Geometry: final body of the model. Coordinates: model frame, mm. Give positions to 0.01 mm unless a question says otherwise; leave off trailing zeros. Order: outer loops, then holes, each group sorted by start corner. A loop starts at its lowest first (then second) coordinate and runs counter-clockwise, first axis right, second up. Notation, with made-up numbers: (25.5, 10) - (56.5, 10) arc R17 ccw to (56.5, 16) - close; hole circle Ø5 at (80, -39). An arc over 180 degrees is marked (long way). One line per item, written item: value.
```python
from build123d import *

# Parameters (mm, degrees)
SKETCH1_W            = 20.5
SKETCH1_H            = 18.5
BOSS_EXTRUDE1_DEPTH  = 2
SKETCH2_W            = 2
SKETCH2_H            = 18.5
BOSS_EXTRUDE2_DEPTH  = 45
SKETCH4_W            = 20.5
SKETCH4_H            = 18.5
BOSS_EXTRUDE3_DEPTH  = 2
SKETCH3_R            = 1.25
CUT_EXTRUDE1_DEPTH   = 50
LPATTERN1_COUNT      = 3
LPATTERN1_PITCH      = 6
LPATTERN1_COUNT_DIR2 = 3
LPATTERN1_PITCH_DIR2 = 6


with BuildPart() as part:
    # Sketch1 → Boss-Extrude1 (new body)
    with BuildSketch(Plane(origin=(0, 0, 0), x_dir=(1, 0, 0), z_dir=(0, 1, 0))):
        Rectangle(SKETCH1_W, SKETCH1_H)
    extrude(amount=BOSS_EXTRUDE1_DEPTH)

    # Sketch2 → Boss-Extrude2 (add)
    with BuildSketch(Plane(origin=(0, 2, 0), x_dir=(1, 0, 0), z_dir=(0, 1, 0))):
        with Locations((9.25, 0)):
            Rectangle(SKETCH2_W, SKETCH2_H)
    extrude(amount=BOSS_EXTRUDE2_DEPTH)

    # Sketch4 → Boss-Extrude3 (add)
    with BuildSketch(Plane(origin=(0, 47, 0), x_dir=(1, 0, 0), z_dir=(0, 1, 0))):
        Rectangle(SKETCH4_W, SKETCH4_H)
    extrude(amount=BOSS_EXTRUDE3_DEPTH)

    # Sketch3 → Cut-Extrude1 (cut, through all)
    with BuildSketch(Plane.XZ):
        with Locations((-7.25, 6.25)):
            Circle(SKETCH3_R)
    cut_extrude1 = extrude(amount=-CUT_EXTRUDE1_DEPTH, mode=Mode.SUBTRACT)

    # LPattern1: Cut-Extrude1 3 × 3
    with Locations(*[(j * LPATTERN1_PITCH_DIR2, 0, -i * LPATTERN1_PITCH) for i in range(LPATTERN1_COUNT) for j in range(LPATTERN1_COUNT_DIR2) if (i, j) != (0, 0)]):
        add(cut_extrude1, mode=Mode.SUBTRACT)


solid = part.part
```
1) Material intervals for line 1 along Z through (x, y) = (4.75, 48.05); line 2 along Y through (x, z) = (-2.75, -7.5); line 3 along X through (y, z) = (22.5, 7), sorted ascending.
Answers below:
line 1: -9.25 to -7, -4.5 to -1, 1.5 to 5, 7.5 to 9.25
line 2: 0 to 2, 47 to 49
line 3: 8.25 to 10.25
2) Section D-D, the plane z = 3.75. Return loops of the section in (x, y).
Answers below:
outline: (-10.25, 0) - (10.25, 0) - (10.25, 49) - (-10.25, 49) - (-10.25, 47) - (8.25, 47) - (8.25, 2) - (-10.25, 2) - close
3) Mould query, pull axis X, two halves, no side actions, for faces 1 (the face through (-1.52, 0.99, 5.03)), 2 (the face through (-1, 47, -2)), 3 (the face through (10.25, 24, 0)), 4 (the face through (-10.25, 48, 0)). Classes: released by +X, released by -X, zero draft, split by the parting line, or undercut.
Answers below:
face 1: undercut
face 2: zero draft
face 3: released by +X
face 4: released by -X
4) First-contact query: pin 1 (4 mm diameter, centred on x = -7.25, z = 6.25, fed in from +Y); pin 2 (4 mm diameter, centred on y = 40, z = 1, fed in from -X). Flat tips, straight axial feed; report the tip coordinate or a pass-through.
Answers below:
pin 1: y = 49
pin 2: x = 8.25
5) Section A-A, the plane z = -0.5. Count the separate pieces of the cut face and the enclosed holes in it, then the cut area to 3 significant figures.
Answers below:
separate pieces: 7
enclosed holes: 0
area: 148 mm^2
6) Section B-B, the plane x = -5. Return loops of the section in (y, z), then the cut area to 3 significant figures.
Answers below:
outline: (0, -9.25) - (2, -9.25) - (2, 9.25) - (0, 9.25) - close; (47, -9.25) - (49, -9.25) - (49, 9.25) - (47, 9.25) - close
area: 74.0 mm^2
